```python
from build123d import *

# Parameters (mm, degrees)
ESTRUSIONE_ESTRUSIONE1_DEPTH = 7.62
CORPO_SPOSTA_COPIA8_ANGLE    = 180
ESTRUSIONE_ESTRUSIONE4_START = -25.4
SCHIZZO11_R                  = 9.5
ESTRUSIONE_ESTRUSIONE4_DEPTH = 146.05
RIPETIZIONE_A_L1_COUNT       = 3
RIPETIZIONE_A_L1_PITCH       = 146.05
CORPO_SPOSTA_COPIA9_ANGLE    = 120
CORPO_SPOSTA_COPIA10_ANGLE   = 120
SCHIZZO12_R                  = 9.5
ESTRUSIONE_ESTRUSIONE5_DEPTH = 24.97


with BuildPart() as part:
    # Schizzo4 → Estrusione-Estrusione1 (new body)
    with BuildSketch(Plane.XY):
        with BuildLine():
            Line((5.499261314, 15.875), (10.998522628, 6.35))
            ThreePointArc((10.998522628, 6.35), (0, -12.7), (-10.998522628, 6.35))
            Line((-10.998522628, 6.35), (-5.499261314, 15.875))
            ThreePointArc((-5.499261314, 15.875), (0, 19.05), (5.499261314, 15.875))
        make_face()
    extrude(amount=ESTRUSIONE_ESTRUSIONE1_DEPTH)


with BuildPart() as body_2:
    # Corpo-Sposta/copia7: copy of part
    add(part.part.moved(Location((0, 0, 60.96))))


with BuildPart() as body_2_1:
    # Corpo-Sposta/copia8: moved
    add(body_2.part.rotate(Axis((0, 0, 0), (0, 0, 1)), CORPO_SPOSTA_COPIA8_ANGLE))


with BuildPart() as part_1:
    add(part.part)

    add(body_2_1.part)  # Estrusione-Estrusione4 merges body 2
    # Schizzo11 → Estrusione-Estrusione4 (add)
    with BuildSketch(Plane.XY.offset(ESTRUSIONE_ESTRUSIONE4_START)):
        Circle(SCHIZZO11_R)
    extrude(amount=ESTRUSIONE_ESTRUSIONE4_DEPTH)


with BuildPart() as ripetizione_a_l1_1:
    # Ripetizione a L1: pattern copy
    add(part_1.part.moved(Location(Vector(0, 0, -1) * (1 * RIPETIZIONE_A_L1_PITCH))))


with BuildPart() as ripetizione_a_l1_2:
    # Ripetizione a L1: pattern copy
    add(part_1.part.moved(Location(Vector(0, 0, -1) * (2 * RIPETIZIONE_A_L1_PITCH))))


with BuildPart() as ripetizione_a_l1_1_1:
    # Corpo-Sposta/copia9: moved
    add(ripetizione_a_l1_1.part.rotate(Axis((0, 0, 0), (0, 0, 1)), CORPO_SPOSTA_COPIA9_ANGLE))


with BuildPart() as ripetizione_a_l1_2_1:
    # Corpo-Sposta/copia10: moved
    add(ripetizione_a_l1_2.part.rotate(Axis((0, 0, 0), (0, 0, -1)), CORPO_SPOSTA_COPIA10_ANGLE))


with BuildPart() as part_2:
    add(part_1.part)

    # Schizzo12 → Estrusione-Estrusione5 (add)
    with BuildSketch(Plane.XY.offset(120.65)):
        Circle(SCHIZZO12_R)
    extrude(amount=ESTRUSIONE_ESTRUSIONE5_DEPTH)


with BuildPart() as ripetizione_a_l1_2_2:
    add(ripetizione_a_l1_2_1.part)

    # Abbina1: union Ripetizione a L1_1, part
    add(ripetizione_a_l1_1_1.part)
    add(part_2.part)


solid = ripetizione_a_l1_2_2.part
```
Input: part model. Units: mm. Frame: model coordinates. A direction names the side the tool comes from. Round coordinates to 2 decimals unless told otherwise and drop trailing zeros. Order: outer loops, then holes, each group sorted by start corner. A loop starts at its lowest first (then second) coordinate and runs counter-clockwise, first axis right, second up. Notation, with made-up numbers: (74.25, 24) - (122.25, 24) arc R16 ccw to (122.25, 35) - close; hole circle Ø5 at (-37, -8). An arc over 180 degrees is marked (long way). Answer in a Markdown table with one row per item.
Item 1: Mould query, pull axis Z, two halves, no side actions, for faces 1 (the flat face through (-1, 10, 7.62)), 2 (the flat face through (-8.2, -11.2, 64.7)), 3 (the flat face through (0, 0, 145.62)). Classes: released by +Z, released by -Z, zero draft, split by the parting line, or undercut.
Model answer:
| item | result |
|---|---|
| face 1 | undercut |
| face 2 | zero draft |
| face 3 | released by +Z |
Item 2: Pin query (flat end, axial travel): pin 1 (2 mm diameter, centred on y = -0.5, z = -223.5, fed in from -X); pin 2 (8 mm diameter, centred on x = -8, z = -187.5, fed in from -Y); pin 3 (6 mm diameter, centred on x = -0.5, y = -10.5, fed in from -Z); pin 4 (4 mm diameter, centred on x = -5, z = 98, fed in from +Y). Return the tip coordinate at first contact, or that it passes through.
Model answer:
| item | result |
|---|---|
| pin 1 | stops at x = -14.95 |
| pin 2 | stops at y = -8.62 |
| pin 3 | stops at z = -317.5 |
| pin 4 | stops at y = 9.01 |
Item 3: Section query A-A (z = -278). Return the cut outline in (x, y), then the cut area to 3 significant figures.
Model answer:
| item | result |
|---|---|
| outline | circle Ø19 at (0, 0) |
| area | 284 mm² |
Item 4: Reachability of faces 4 (the cylindrical face through (-0.372, 12.695, 64.717)), 5 (the flat face through (13.71, 1.65, -288.34)), 6 (the cylindrical face through (-2.059, -9.274, -304.978)), 7 (the flat face through (-7, -7, -138.43)), 8 (the flat face through (-5, -12.7, -142)) from +Z, -Z, +X, -X, +Y, -Y: full face, straight path, thin tool, end or side. Return the list, or none.
Model answer:
| item | result |
|---|---|
| face 4 | +Z |
| face 5 | -Z, +X, +Y |
| face 6 | -Z |
| face 7 | none |
| face 8 | -Z, +X, -X, -Y |
Item 5: Line query: line 1 (Z direction, x = -11, y = 6); line 2 (Z direction, x = 13.5, y = 0); line 3 (Z direction, x = 5, y = -15). Output: solid intervals per line, ascending.
Model answer:
| item | result |
|---|---|
| line 1 | z = -292.1 to -284.48, -231.14 to -223.52, -146.05 to -138.43, -85.09 to -77.47, 0 to 7.62, 60.96 to 68.58 |
| line 2 | z = -292.1 to -284.48, -85.09 to -77.47 |
| line 3 | z = 60.96 to 68.58 |
